Could you check a few things on this model? Use its own coordinates, in mm. A direction names the side the tool comes from. Coordinates: 2 decimals unless noted, no trailing zeros. Order: outer loops, then holes, each group sorted by start corner. A loop starts at its lowest first (then second) coordinate and runs counter-clockwise, first axis right, second up. Notation, with made-up numbers: (-18, -33.75) - (31, -33.75) arc R21 ccw to (31, -11.75) - close; hole circle Ø5 at (-35.5, 32.5). An arc over 180 degrees is marked (long way). Answer as a JSON object with one key per item and string values. Group by question number.
(1) Please list where these lines run through material, in increasing order: probe 1 along Z at (x, y) = (-72.5, 1.75); probe 2 along X at (y, z) = (1.5, 8.5); probe 3 along X at (y, z) = (-0.25, 19).
(2) Will these pins go through, and if not, where does the flat tip stop? P1, Ø2, axis at x = 146.825, z = -15, coming from the +Y side; P2, Ø1.9, axis at x = -100, y = 0, coming from the +Z side.
(3) Imagine slicing it at B-B, the plane z = 9. Write out the boundary of the cut face in (x, y) (3 decimals), and give its area (3 significant figures).
(4) Imagine slicing it at A-A, the plane z = -10. Write out the boundary of the cut face in (x, y) (3 decimals).
(5) Which directions (+Z, -Z, +X, -X, +Y, -Y) give clear straight access to the entire face, cutting with the end or side of a thin tool? Please do faces 4 (the flat face through (-117, 0, -14)), 5 (the flat face through (-2, 0, -25)).
(6) We'd pull the mould along X, two halves only. Please class faces 1 (the flat face through (-140, 0, 0)), 2 (the flat face through (-2, 0, 25)), 3 (the flat face through (150, 0, 0)): pulls with the +X half, pulls with the -X half, needs draft (parallel to the pull), parting line crosses it, or undercut.
from build123d import *

# Parameters (mm, degrees)
F0_W     = 300
F0_H     = 50
F0_W_2   = 47.5
F0_H_2   = 28
F0_R     = 5
F1_DEPTH = 3.175
F3_D     = 2.4
F5_D     = 2.4
F5_DEPTH = 12
F5_TIP   = 0.7210327428
F7_D     = 5.5


with BuildPart() as f1:
    # F0 (on Front) → F1 (new body, symmetric)
    with BuildSketch(Plane.XZ):
        Rectangle(F0_W, F0_H)
        with Locations((-116.25, 0)):
            Rectangle(F0_W_2, F0_H_2, mode=Mode.SUBTRACT)
        with Locations((-72.5, 9)):
            Circle(F0_R, mode=Mode.SUBTRACT)
    extrude(amount=F1_DEPTH, both=True)

    # F3 (through all)
    with Locations(Plane.XZ.offset(3.175)):
        with Locations((-146.825, 15), (-146.825, -15), (146.825, 15), (146.825, -15)):
            Hole(F3_D / 2)

    # F5
    with Locations(Plane.XY.offset(25)):
        with Locations((-100, 0), (100, 0)):
            Hole(F5_D / 2, depth=F5_DEPTH)
            with Locations((0, 0, -(F5_DEPTH + F5_TIP / 2))):  # 118° drill point
                Cone(0, F5_D / 2, F5_TIP, mode=Mode.SUBTRACT)

    # F7 (through all)
    with Locations(Plane.XZ.offset(3.175)):
        with Locations((-72.5, -10)):
            Hole(F7_D / 2)


solid = f1.part
Result set:
{
 "1": {"probe 1": "z = -25 to -12.75, -7.25 to 4, 14 to 25", "probe 2": "x = -150 to -140, -92.5 to -77.47, -67.53 to 150", "probe 3": "x = -150 to -101.17, -98.83 to 98.83, 101.17 to 150"},
 "2": {"P1": "passes through", "P2": "stops at z = -14"},
 "3": {"outline": "(-150, -3.175) - (-140, -3.175) - (-140, 3.175) - (-150, 3.175) - close; (-92.5, -3.175) - (-77.5, -3.175) - (-77.5, 3.175) - (-92.5, 3.175) - close; (-67.5, -3.175) - (150, -3.175) - (150, 3.175) - (-67.5, 3.175) - close", "area": "1,540 mm^2"},
 "4": {"outline": "(-150, -3.175) - (-140, -3.175) - (-140, 3.175) - (-150, 3.175) - close; (-92.5, -3.175) - (-75.25, -3.175) - (-75.25, 3.175) - (-92.5, 3.175) - close; (-69.75, -3.175) - (150, -3.175) - (150, 3.175) - (-69.75, 3.175) - close"},
 "5": {"face 4": "+Y, -Y", "face 5": "-Z, +X, -X, +Y, -Y"},
 "6": {"face 1": "undercut", "face 2": "needs draft", "face 3": "pulls with the +X half"}
}
